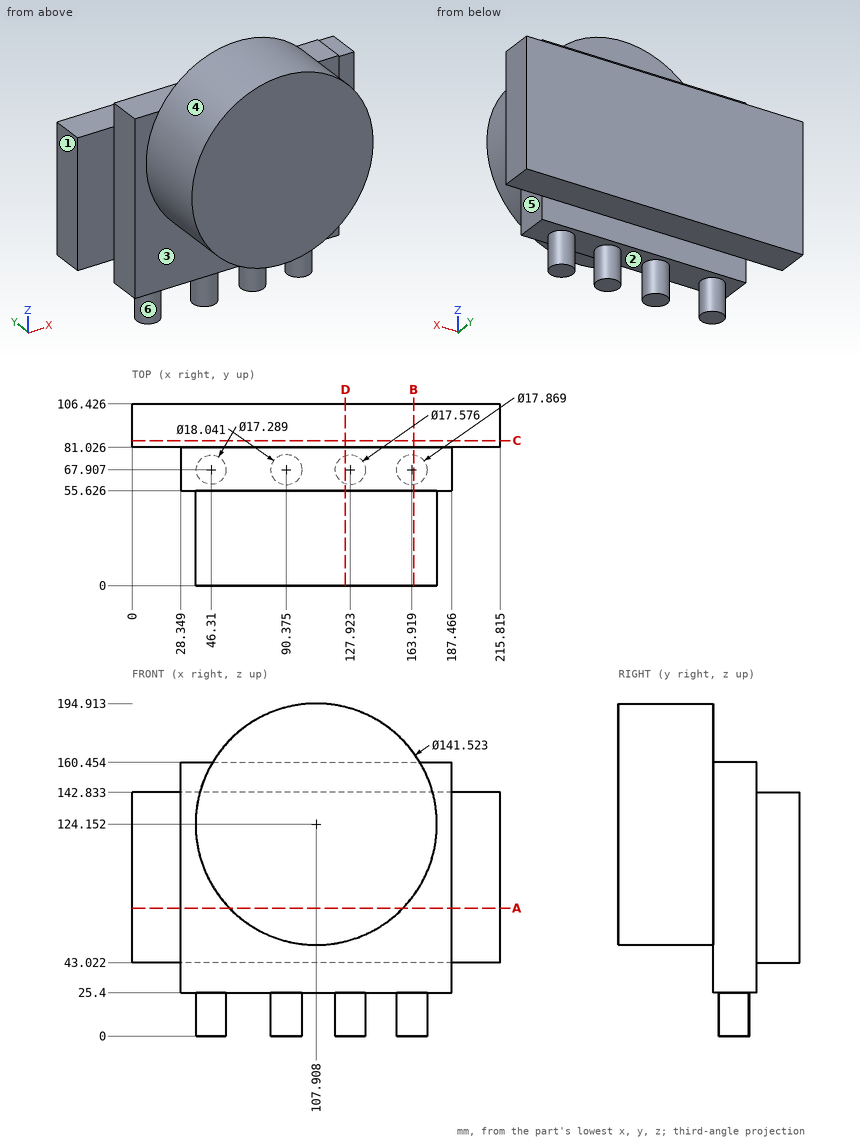
Input: dimensioned drawing with shaded views. Units: mm. Origin: part minimum x, y, z. A direction names the side the tool comes from. Give positions to 0.01 mm unless a question says otherwise; leave off trailing zeros. Write each loop counter-clockwise with the first axis right and the second up, starting at its lowest first coordinate (ties: lowest second). Pieces come first, ordered by that corner, then holes. Notation, with made-up numbers: (-33, 44) -> (-29, 44) arc R13 cw to (-29, 54) -> close; hole circle Ø3 at (-21.5, 55.5). An arc over 180 degrees is marked (long way). Answer as a JSON object with one key per item and string values.
1. Cut plane A-A on z = 75. Output: boundary loops of the cut face in (x, y) (1 decimal).
Ans:
{"outline": "(0, 81) -> (28.3, 81) -> (28.3, 55.6) -> (57, 55.6) -> (57, 0) -> (158.8, 0) -> (158.8, 55.6) -> (187.5, 55.6) -> (187.5, 81) -> (215.8, 81) -> (215.8, 106.4) -> (0, 106.4) -> close"}
2. Ray query, probe 1 along X at (y, z) = (68.5, 32.5); probe 2 along Z at (x, y) = (88, 93); probe 3 along Y at (x, z) = (166.5, 155) (1 decimal). Return the intervals inside material, ascending. Write a range as from..to.
Ans:
{"probe 1": "x = 28.35..187.47", "probe 2": "z = 43.02..142.83", "probe 3": "y = 0..81"}
3. Mould query, pull axis X, two halves, no side actions, for the marked faces 1, 2 and 3. Classes: pulls with the +X half, pulls with the -X half, needs draft (parallel to the pull), parting line crosses it, or undercut.
Ans:
{"face 1": "pulls with the -X half", "face 2": "undercut", "face 3": "needs draft"}
4. Cut plane D-D on x = 125. Output: boundary loops of the cut face in (y, z) (1 decimal), and give its area (3 significant figures).
Ans:
{"outline": "(0, 55.5) -> (55.6, 55.5) -> (55.6, 25.4) -> (59.6, 25.4) -> (59.6, 0) -> (76.2, 0) -> (76.2, 25.4) -> (81, 25.4) -> (81, 43) -> (106.4, 43) -> (106.4, 142.8) -> (81, 142.8) -> (81, 160.5) -> (55.6, 160.5) -> (55.6, 192.8) -> (0, 192.8) -> close", "area": "14,000 mm^2"}
5. Cut plane C-C on y = 85. Output: boundary loops of the cut face in (x, z) (1 decimal), and give its area (3 significant figures).
Ans:
{"outline": "(0, 43) -> (215.8, 43) -> (215.8, 142.8) -> (0, 142.8) -> close", "area": "21,500 mm^2"}
6. Access query for the marked faces 4, 5 and 6. Directions: +Z, -Z, +X, -X, +Y, -Y. A direction counts if a zero-diameter tool reaches every point of the face in a straight line with its end or side. Return the directions, or none.
Ans:
{"face 4": "-Y", "face 5": "+Z, -Z, +X, -Y", "face 6": "-Z"}
7. Contact query for flat-ended pins moving along their axis: pin 1 (5 mm diameter, centred on x = 34, y = 57.5, fed in from -Z); pin 2 (20.5 mm diameter, centred on y = 69, z = 119, fed in from -X); pin 3 (8 mm diameter, centred on x = 135.5, y = 17, fed in from -Z). Output: stop coordinate, or through.
Ans:
{"pin 1": "stops at z = 25.4", "pin 2": "stops at x = 28.35", "pin 3": "stops at z = 57.44"}
8. Cut plane B-B on x = 165. Output: boundary loops of the cut face in (y, z) (1 decimal), and give its area (3 significant figures).
Ans:
{"outline": "(0, 82.3) -> (55.6, 82.3) -> (55.6, 25.4) -> (59, 25.4) -> (59, 0) -> (76.8, 0) -> (76.8, 25.4) -> (81, 25.4) -> (81, 43) -> (106.4, 43) -> (106.4, 142.8) -> (81, 142.8) -> (81, 160.5) -> (55.6, 160.5) -> (55.6, 166) -> (0, 166) -> close", "area": "11,100 mm^2"}
